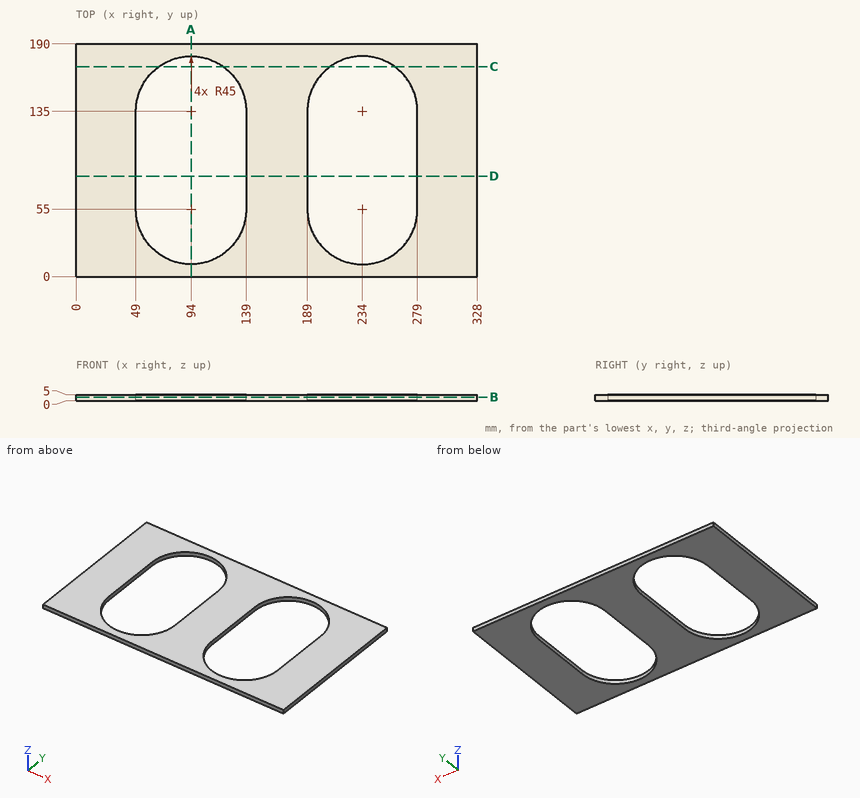
Drawing for the job (mm, zero at the part's lowest x, y, z). Give positions to 0.01 mm unless a question says otherwise; leave off trailing zeros. Order: outer loops, then holes, each group sorted by start corner. A loop starts at its lowest first (then second) coordinate and runs counter-clockwise, first axis right, second up. Notation, with made-up numbers: M 9,48 L 68,48 A28 ccw 68,86 Z; hole C 61,-26 d11. An arc over 180 degrees is marked long. Put each result on its own line as item: value. Start each with the question number.
(1) Saw through at B-B, the plane z = 2.9. Write the cut outline in (x, y).
(2) Saw through at C-C, the plane y = 171.5. Write the cut outline in (x, z), then the cut area to 3 significant figures.
(3) Drill centre lines: line 1 along X through (y, z) = (104, 2.65); line 2 along X through (y, z) = (166, 4.15); line 3 along Y through (x, z) = (236, 0.95). Where is each one in solid material? Low to high.
(4) Saw through at D-D, the plane y = 82. Write the cut outline in (x, z).
(5) Saw through at A-A, the plane x = 94. Write the cut outline in (y, z), then the cut area to 3 significant figures.
Check result:
1. outline: M 0,0 L 328,0 L 328,190 L 0,190 Z; hole M 49,55 A45 ccw 139,55 L 139,135 A45 ccw 49,135 Z; hole M 189,55 A45 ccw 279,55 L 279,135 A45 ccw 189,135 Z
2. outline: M 0,0 L 67.68,0 L 67.68,5 L 0,5 Z; M 120.32,0 L 207.68,0 L 207.68,5 L 120.32,5 Z; M 260.32,0 L 328,0 L 328,5 L 260.32,5 Z
2. area: 1,110 mm2
3. line 1: x = 0 to 49, 139 to 189, 279 to 328
3. line 2: x = 0 to 61.38, 126.62 to 201.38, 266.62 to 328
3. line 3: y = 0 to 10.04, 179.96 to 190
4. outline: M 0,0 L 49,0 L 49,5 L 0,5 Z; M 139,0 L 189,0 L 189,5 L 139,5 Z; M 279,0 L 328,0 L 328,5 L 279,5 Z
5. outline: M 0,0 L 10,0 L 10,5 L 0,5 Z; M 180,0 L 190,0 L 190,5 L 180,5 Z
5. area: 100 mm2
